Verification items for the finished model (mm, model axes). Coordinates: 2 decimals unless noted, no trailing zeros. Order: outer loops, then holes, each group sorted by start corner. A loop starts at its lowest first (then second) coordinate and runs counter-clockwise, first axis right, second up. Notation, with made-up numbers: (30, -34) -> (41, -34) arc R20 cw to (41, -26) -> close; hole circle Ø3 at (-37.75, 82). An arc over 180 degrees is marked (long way). Write item = value, one per line. Start each with the question number.
1. Thickness scan on line 1 along Y through (x, z) = (224, 1.3); line 2 along Y through (x, z) = (393, 0.95); line 3 along X through (y, z) = (37, 1.25). Record the ranges inside material, lowest first. Write a range as from..to.
2. Go/stop test with flat-tipped pins: P1, Ø0.8, axis at x = 146, z = 1, coming from the -Y side; P2, Ø0.6, axis at y = 27, z = 1, coming from the +X side; P3, Ø5, axis at x = 403, y = 14, coming from the +Z side; P4, Ø0.7, axis at x = 416.5, z = 1, coming from the +Y side. Record where each tip stops, or that it passes through.
3. Cross-section at B-B on z = 0.3. Give the number of separate pieces and of enclosed holes in the cut face, plus the area to 3 significant figures.
4. Cross-section at A-A on x = 127. Record the cut outline in (y, z).
from build123d import *

# Parameters (mm, degrees)
SKETCH_1_W      = 1.499999968
SKETCH_1_H      = 6.000000011
SKETCH_1_H_2    = 6.00000001
SKETCH_1_W_2    = 1.5
SKETCH_1_H_3    = 6
EXTRUDE_1_DEPTH = 2


with BuildPart() as part:
    # 草图1 → 凸台-拉伸1 (new body)
    with BuildSketch(Plane.XY):
        Polygon((537.351209242, 34.194218327), (539.351209242, 34.194218327), (539.351209242, 28.194218337), (537.351209274, 28.194218337), (537.351209274, 21.391410378), (11.364676515, 10.534074896), (11.364676515, 38.388326082), (537.351216266, 40.712891717), align=None)
        with Locations((416.371863849, 29.143567663)):
            Rectangle(SKETCH_1_W, SKETCH_1_H, mode=Mode.SUBTRACT)
        with Locations((286.128813818, 28.050804453)):
            Rectangle(SKETCH_1_W, SKETCH_1_H_2, mode=Mode.SUBTRACT)
        with Locations((145.867074626, 26.415625273)):
            Rectangle(SKETCH_1_W_2, SKETCH_1_H_3, mode=Mode.SUBTRACT)
        Polygon((531.351209242, 34.686316456), (531.351209242, 27.268837395), (497.351863833, 26.567027983), (497.351863833, 34.536058409), align=None, mode=Mode.SUBTRACT)
        Polygon((493.351863833, 26.48446058), (461.121863833, 25.819173732), (461.121863833, 34.37594212), (493.351863833, 34.518380652), align=None, mode=Mode.SUBTRACT)
        Polygon((457.121863833, 25.736606329), (423.121863833, 25.034783405), (423.121863833, 34.208003423), (457.121863833, 34.358264363), align=None, mode=Mode.SUBTRACT)
        Polygon((409.621863833, 34.148340991), (409.621863833, 24.75611842), (372.718813802, 23.994371171), (372.718813802, 33.985250198), align=None, mode=Mode.SUBTRACT)
        Polygon((368.718813802, 23.911803768), (333.778813802, 23.190577505), (333.778813802, 33.813157228), (368.718813802, 33.967572441), align=None, mode=Mode.SUBTRACT)
        Polygon((329.778813802, 23.108010102), (292.878813802, 22.346325811), (292.878813802, 33.632402157), (329.778813802, 33.79547947), align=None, mode=Mode.SUBTRACT)
        Polygon((279.378813802, 33.572739725), (279.378813802, 22.067660826), (239.377074626, 21.241950898), (239.377074626, 33.395954463), align=None, mode=Mode.SUBTRACT)
        Polygon((235.377074626, 21.159383496), (196.617074626, 20.359305362), (196.617074626, 33.206979234), (235.377074626, 33.378276705), align=None, mode=Mode.SUBTRACT)
        Polygon((192.617074626, 20.276737959), (152.617074626, 19.451063931), (152.617074626, 33.012523901), (192.617074626, 33.189301477), align=None, mode=Mode.SUBTRACT)
        Polygon((139.117074626, 32.952861469), (139.117074626, 19.172398947), (101.114676515, 18.387959118), (101.114676515, 32.784912174), align=None, mode=Mode.SUBTRACT)
        Polygon((97.114676515, 18.305391716), (59.364676515, 17.526161852), (59.364676515, 32.600400579), (97.114676515, 32.767234416), align=None, mode=Mode.SUBTRACT)
        Polygon((55.364676515, 17.443594449), (17.364676515, 16.659204122), (17.364676515, 32.414784125), (55.364676515, 32.582722822), align=None, mode=Mode.SUBTRACT)
    extrude(amount=EXTRUDE_1_DEPTH)


solid = part.part
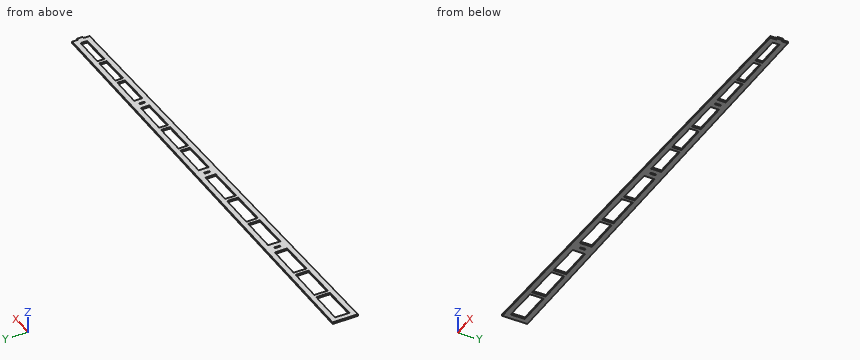
Worked out:
q1.line_1 = 14.92..20.92, 33.33..39.33
q1.line_2 = 18.41..24.41, 34.07..40.07
q1.line_3 = 11.36..537.35
q2.P1 = 13.3
q2.P2 = 537.35
q2.P3 = through
q2.P4 = 40.18
q3.separate_pieces = 1
q3.enclosed_holes = 15
q3.area = 7,270 mm²
q4.outline = (12.92, 0) -> (18.92, 0) -> (18.92, 2) -> (12.92, 2) -> close; (32.9, 0) -> (38.9, 0) -> (38.9, 2) -> (32.9, 2) -> close
